Input: part model. Units: mm. Frame: model coordinates. A direction names the side the tool comes from. Give positions to 0.01 mm unless a question says otherwise; leave off trailing zeros. Write each loop counter-clockwise with the first axis right and the second up, starting at its lowest first coordinate (ties: lowest second). Pieces come first, ordered by that corner, then holes. Notation, with made-up numbers: (86, -35.75) - (115, -35.75) arc R8 ccw to (115, -25.75) - close; hole circle Ø10 at (29.5, -37). An arc over 180 degrees is marked (long way). Use a Markdown table: item, result. Add a question column.
1. Pin query (flat end, axial travel): pin 1 (1.5 mm diameter, centred on x = 26, y = -238, fed in from -Z); pin 2 (3 mm diameter, centred on y = -254, z = -30.48, fed in from +X); pin 3 (0.6 mm diameter, centred on x = -26, z = -51, fed in from +Y). Return the tip coordinate at first contact, or that it passes through.
2. Section query A-A, the plane y = -432. Return loops of the section in (x, z), plus the area to 3 significant figures.
3. Mould query, pull axis X, two halves, no side actions, for faces 1 (the flat face through (0, -546.1, -1)), 2 (the flat face through (26.678, 114, -33)), 3 (the flat face through (0, 8, -1.897)). Classes: released by +X, released by -X, zero draft, split by the parting line, or undercut.
4. Section query B-B, the plane x = -1.5. Return loops of the section in (y, z), plus the area to 3 significant figures.
5. Set-up query: faces 4 (the flat face through (-26.678, 129, -33)), 5 (the flat face through (-24.78, 129, -33)). Return all of +Z, -Z, +X, -X, +Y, -Y with unobstructed straight access to the full face (end or side cutting, diameter ignored); none if empty.
6. Material intervals for probe 1 along Y at (x, z) = (25.65, -63.5) (3 decimals); probe 2 along X at (y, z) = (15, -36); probe 3 along Z at (x, y) = (20, 14), sorted ascending.
```python
from build123d import *

# Parameters (mm, degrees)
SKETCH1_W                    = 53.35524
SKETCH1_H                    = 1092.2
BASE_FLANGE1_DEPTH           = 1.89738
EDGE_FLANGE1_STRIP_W         = 11.65352
EDGE_FLANGE1_STRIP_H         = 1.89738
EDGE_FLANGE1_STRIP_CUT_DEPTH = 1092.2
EDGE_FLANGE1_DEPTH           = 1092.2
EDGE_FLANGE1_FLAT_DEPTH      = 1.89738
EDGE_FLANGE2_STRIP_W         = 11.65352
EDGE_FLANGE2_STRIP_H         = 1.89738
EDGE_FLANGE2_STRIP_CUT_DEPTH = 1092.2
EDGE_FLANGE2_DEPTH           = 1092.2
EDGE_FLANGE2_FLAT_DEPTH      = 1.89738
FILLET1_R                    = 2.54
SKETCH12_R                   = 2.4638
CUT_EXTRUDE1_DEPTH           = 554.966092496
SKETCH13_R                   = 2.4638
CUT_EXTRUDE2_DEPTH           = 554.966092496
SKETCH14_R                   = 2.4638
CUT_EXTRUDE3_DEPTH           = 554.966092496
E_0_25_DIAMETER_HOLE1_D      = 6.35


# Sheet-metal steps are written as plain solids
with BuildPart() as part:
    # Sketch1 → Base-Flange1 (new body)
    with BuildSketch(Plane.XY):
        Rectangle(SKETCH1_W, SKETCH1_H)
    extrude(amount=-BASE_FLANGE1_DEPTH)

    # Edge-Flange1 strip (across the edge) → Edge-Flange1 strip cut (cut)
    with BuildSketch(Plane(origin=(26.67762, 546.1, -1.89738), x_dir=(-1, 0, 0), z_dir=(0, -1, 0))):
        with Locations((-1.89738, -0.94869)):
            Rectangle(EDGE_FLANGE1_STRIP_W, EDGE_FLANGE1_STRIP_H)
    extrude(amount=EDGE_FLANGE1_STRIP_CUT_DEPTH, mode=Mode.SUBTRACT)

    # Edge-Flange1 bend section (across the edge) → Edge-Flange1 (add)
    with BuildSketch(Plane(origin=(26.67762, 546.1, -1.89738), x_dir=(-1, 0, 0), z_dir=(0, -1, 0))):
        with BuildLine():
            Line((0, 2.032), (1.89738, 2.032))
            ThreePointArc((1.89738, 2.032), (2.492539021, 0.595159021), (3.92938, 0))
            Line((3.92938, 0), (3.92938, -1.89738))
            ThreePointArc((3.92938, -1.89738), (1.150888756, -0.746491244), (0, 2.032))
        make_face()
    extrude(amount=EDGE_FLANGE1_DEPTH)

    # Edge-Flange1 profile (on flange) → Edge-Flange1 flat (add)
    with BuildSketch(Plane(origin=(26.67762, 0, -1.89738), x_dir=(0, 1, 0), z_dir=(-1, 0, 0))):
        with BuildLine():
            Line((540.223938633, 36.20262), (441.325, 36.20262))
            ThreePointArc((441.325, 36.20262), (439.07993597, 37.13255597), (438.15, 39.37762))
            Line((438.15, 39.37762), (438.15, 71.12762))
            ThreePointArc((438.15, 71.12762), (437.22006403, 73.37268403), (434.975, 74.30262))
            Line((434.975, 74.30262), (-9.525, 74.30262))
            ThreePointArc((-9.525, 74.30262), (-11.77006403, 73.37268403), (-12.7, 71.12762))
            Line((-12.7, 71.12762), (-12.7, 39.37762))
            ThreePointArc((-12.7, 39.37762), (-13.62993597, 37.13255597), (-15.875, 36.20262))
            Line((-15.875, 36.20262), (-546.1, 36.20262))
            Line((-546.1, 36.20262), (-546.1, 2.032))
            Line((-546.1, 2.032), (546.1, 2.032))
            Line((546.1, 2.032), (546.1, 2.87782))
            Line((546.1, 2.87782), (540.223938633, 36.20262))
        make_face()
    extrude(amount=EDGE_FLANGE1_FLAT_DEPTH)

    # Edge-Flange2 strip (across the edge) → Edge-Flange2 strip cut (cut)
    with BuildSketch(Plane(origin=(-26.67762, -546.1, -1.89738), x_dir=(1, 0, 0), z_dir=(0, 1, 0))):
        with Locations((-1.89738, -0.94869)):
            Rectangle(EDGE_FLANGE2_STRIP_W, EDGE_FLANGE2_STRIP_H)
    extrude(amount=EDGE_FLANGE2_STRIP_CUT_DEPTH, mode=Mode.SUBTRACT)

    # Edge-Flange2 bend section (across the edge) → Edge-Flange2 (add)
    with BuildSketch(Plane(origin=(-26.67762, -546.1, -1.89738), x_dir=(1, 0, 0), z_dir=(0, 1, 0))):
        with BuildLine():
            Line((0, 2.032), (1.89738, 2.032))
            ThreePointArc((1.89738, 2.032), (2.492539021, 0.595159021), (3.92938, 0))
            Line((3.92938, 0), (3.92938, -1.89738))
            ThreePointArc((3.92938, -1.89738), (1.150888756, -0.746491244), (0, 2.032))
        make_face()
    extrude(amount=EDGE_FLANGE2_DEPTH)

    # Edge-Flange2 profile (on flange) → Edge-Flange2 flat (add)
    with BuildSketch(Plane(origin=(-26.67762, 0, -1.89738), x_dir=(0, -1, 0), z_dir=(1, 0, 0))):
        with BuildLine():
            Line((-441.325, 36.20262), (-540.223938633, 36.20262))
            Line((-540.223938633, 36.20262), (-546.1, 2.87782))
            Line((-546.1, 2.87782), (-546.1, 2.032))
            Line((-546.1, 2.032), (546.1, 2.032))
            Line((546.1, 2.032), (546.1, 36.20262))
            Line((546.1, 36.20262), (15.875, 36.20262))
            ThreePointArc((15.875, 36.20262), (13.62993597, 37.13255597), (12.7, 39.37762))
            Line((12.7, 39.37762), (12.7, 71.12762))
            ThreePointArc((12.7, 71.12762), (11.77006403, 73.37268403), (9.525, 74.30262))
            Line((9.525, 74.30262), (-434.975, 74.30262))
            ThreePointArc((-434.975, 74.30262), (-437.22006403, 73.37268403), (-438.15, 71.12762))
            Line((-438.15, 71.12762), (-438.15, 39.37762))
            ThreePointArc((-438.15, 39.37762), (-439.07993597, 37.13255597), (-441.325, 36.20262))
        make_face()
    extrude(amount=EDGE_FLANGE2_FLAT_DEPTH)

    # Fillet1
    fillet1_edges = [part.edges().sort_by_distance(p)[0] for p in [
        (25.72893, -546.1, -38.1),
        (25.72893, 540.223938633, -38.1),
        (-25.72893, -546.1, -38.1),
        (-25.72893, 540.223938633, -38.1),
    ]]
    fillet(fillet1_edges, radius=FILLET1_R)

    # Sketch12 → Cut-Extrude1 (cut, through all)
    with BuildSketch(Plane.ZY.offset(26.67762)):
        with Locations((-30.48, -538.48)):
            Circle(SKETCH12_R)
        with Locations((-30.48, -519.43)):
            Circle(SKETCH12_R)
        with Locations((-11.43, -519.43)):
            Circle(SKETCH12_R)
        with Locations((-11.43, -538.48)):
            Circle(SKETCH12_R)
    extrude(amount=-CUT_EXTRUDE1_DEPTH, mode=Mode.SUBTRACT)

    # Sketch13 → Cut-Extrude2 (cut, through all)
    with BuildSketch(Plane.ZY.offset(26.67762)):
        with Locations((-30.48, 533.262579053)):
            Circle(SKETCH13_R)
        with Locations((-11.43, 536.621608035)):
            Circle(SKETCH13_R)
        with Locations((-11.43, 517.277731079)):
            Circle(SKETCH13_R)
        with Locations((-30.48, 513.918702097)):
            Circle(SKETCH13_R)
    extrude(amount=-CUT_EXTRUDE2_DEPTH, mode=Mode.SUBTRACT)

    # Sketch14 → Cut-Extrude3 (cut, through all)
    with BuildSketch(Plane(origin=(26.67762, 0, 0), x_dir=(0, 0, -1), z_dir=(1, 0, 0))):
        with Locations((11.43, -234.95)):
            Circle(SKETCH14_R)
        with Locations((11.43, -254)):
            Circle(SKETCH14_R)
        with Locations((30.48, -254)):
            Circle(SKETCH14_R)
        with Locations((30.48, -234.95)):
            Circle(SKETCH14_R)
    extrude(amount=-CUT_EXTRUDE3_DEPTH, mode=Mode.SUBTRACT)

    # E (0.25) Diameter Hole1 (through all)
    with Locations(Plane(origin=(26.67762, 0, 0), x_dir=(0, 0, -1), z_dir=(1, 0, 0))):
        with Locations((63.5, 415.29), (63.5, 8.89)):
            Hole(E_0_25_DIAMETER_HOLE1_D / 2)


solid = part.part
```
Result sheet:
| question | item | result |
|---|---|---|
| 1 | pin 1 | stops at z = -38.1 |
| 1 | pin 2 | passes through |
| 1 | pin 3 | stops at y = 438.15 |
| 2 | outline | (-26.68, -38.1) - (-24.78, -38.1) - (-24.78, -3.93) arc R2.03 cw to (-22.75, -1.9) - (22.75, -1.9) arc R2.03 cw to (24.78, -3.93) - (24.78, -38.1) - (26.68, -38.1) - (26.68, -3.93) arc R3.93 ccw to (22.75, 0) - (-22.75, 0) arc R3.93 ccw to (-26.68, -3.93) - close |
| 2 | area | 234 mm² |
| 3 | face 1 | zero draft |
| 3 | face 2 | released by +X |
| 3 | face 3 | undercut |
| 4 | outline | (-546.1, -1.9) - (546.1, -1.9) - (546.1, 0) - (-546.1, 0) - close |
| 4 | area | 2,070 mm² |
| 5 | face 4 | +Z, -Z, -X, +Y, -Y |
| 5 | face 5 | -Z, +Y, -Y |
| 6 | probe 1 | y = -12.7 to 5.715, 12.065 to 412.115, 418.465 to 438.15 |
| 6 | probe 2 | x = -26.68 to -24.78, 24.78 to 26.68 |
| 6 | probe 3 | z = -1.9 to 0 |
